Source: CAD feature listing. Evaluate the final solid. Frame: model axes, mm. Face numbers are marked on the shaded views. A direction names the side the tool comes from. Coordinates: 2 decimals unless noted, no trailing zeros. Order: outer loops, then holes, each group sorted by start corner. A loop starts at its lowest first (then second) coordinate and runs counter-clockwise, first axis right, second up. Notation, with made-up numbers: (23, 70.25) - (71, 70.25) arc R3 cw to (71, 74.25) - close; hole circle Ø5 at (64, 30.25). An arc over 180 degrees is marked (long way). One line per question, with ' | ' between items.
from build123d import *

# Parameters (mm, degrees)
BOSS_EXTRUDE1_DEPTH = 15
SKETCH4_R           = 37.5
BOSS_EXTRUDE2_DEPTH = 25
SKETCH5_R           = 22.5
CUT_EXTRUDE1_DEPTH  = 179.290493297
SKETCH6_R           = 32.5
CUT_EXTRUDE2_DEPTH  = 15
SKETCH7_R           = 15
CUT_EXTRUDE3_DEPTH  = 178.165177165
SKETCH9_R           = 15
BOSS_EXTRUDE3_DEPTH = 5
SKETCH10_R          = 1.5
CUT_EXTRUDE7_DEPTH  = 3


with BuildPart() as part:
    # Sketch2 → Boss-Extrude1 (new body)
    with BuildSketch(Plane(origin=(0, 0, 0), x_dir=(1, 0, 0), z_dir=(0, 1, 0))):
        with BuildLine():
            Line((0, 22.5), (150, 22.5))
            ThreePointArc((150, 22.5), (172.5, 0), (150, -22.5))
            Line((150, -22.5), (0, -22.5))
            ThreePointArc((0, -22.5), (-22.5, 0), (0, 22.5))
        make_face()
    extrude(amount=BOSS_EXTRUDE1_DEPTH)

    # Sketch4 → Boss-Extrude2 (add)
    with BuildSketch(Plane(origin=(0, 15, 0), x_dir=(1, 0, 0), z_dir=(0, 1, 0))):
        with Locations(Location((0, 0, 0), (0, 0, 270))):
            Circle(SKETCH4_R)
    extrude(amount=-BOSS_EXTRUDE2_DEPTH)

    # Sketch5 → Cut-Extrude1 (cut, through all)
    with BuildSketch(Plane(origin=(0, 15, 0), x_dir=(1, 0, 0), z_dir=(0, 1, 0))):
        with Locations(Location((0, 0, 0), (0, 0, 270))):
            Circle(SKETCH5_R)
    extrude(amount=-CUT_EXTRUDE1_DEPTH, mode=Mode.SUBTRACT)

    # Sketch6 → Cut-Extrude2 (cut)
    with BuildSketch(Plane(origin=(0, 15, 0), x_dir=(1, 0, 0), z_dir=(0, 1, 0))):
        with Locations(Location((0, 0, 0), (0, 0, 270))):
            Circle(SKETCH6_R)
    extrude(amount=-CUT_EXTRUDE2_DEPTH, mode=Mode.SUBTRACT)

    # Sketch7 → Cut-Extrude3 (cut, through all)
    with BuildSketch(Plane.XZ):
        with Locations(Location((150, 0, 0), (0, 0, 270))):
            Circle(SKETCH7_R)
    extrude(amount=-CUT_EXTRUDE3_DEPTH, mode=Mode.SUBTRACT)

    # Sketch9 → Boss-Extrude3 (add)
    with BuildSketch(Plane.XZ):
        with Locations(Location((150, 0, 0), (0, 0, 270))):
            Circle(SKETCH9_R)
    extrude(amount=-BOSS_EXTRUDE3_DEPTH)

    # Sketch10 → Cut-Extrude7 (cut)
    with BuildSketch(Plane(origin=(0, 15, 0), x_dir=(1, 0, 0), z_dir=(0, 1, 0))):
        with Locations(Location((0, -34.5, 0), (0, 0, 270))):
            Circle(SKETCH10_R)
        with Locations(Location((34.5, 0, 0), (0, 0, 270))):
            Circle(SKETCH10_R)
        with Locations(Location((0, 34.5, 0), (0, 0, 270))):
            Circle(SKETCH10_R)
    extrude(amount=-CUT_EXTRUDE7_DEPTH, mode=Mode.SUBTRACT)


solid = part.part
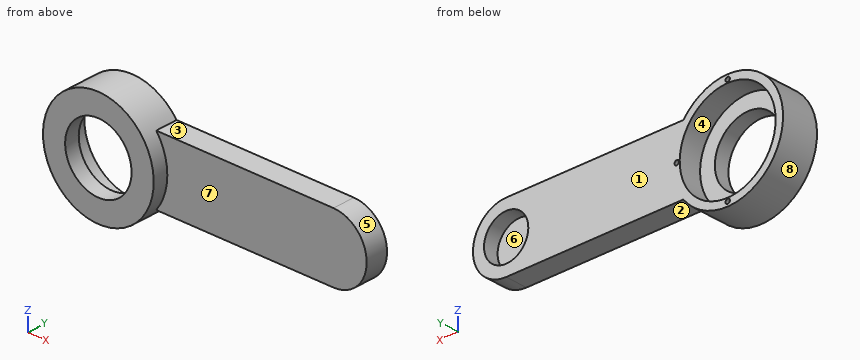
(1) Pin query (flat end, axial travel): P1, Ø12, axis at x = 84, y = 8, coming from the -Z side; P2, Ø3.5, axis at x = -0.5, z = 34.5, coming from the +Y side; P3, Ø22.5, axis at x = 91.5, z = -11, coming from the -Y side; P4, Ø1.5, axis at y = -6, z = 26, coming from the +X side. Return the tip coordinate at first contact, or that it passes through.
Taken from the geometry:
P1: stops at z = -22.5 | P2: stops at y = 15 | P3: stops at y = 0 | P4: stops at x = 27.73
(2) Pull-direction query (X, two-part tool) for the marked faces 6, 7 and 8; classes: pulls with the +X half, pulls with the -X half, needs draft (parallel to the pull), parting line crosses it, or undercut.
Taken from the geometry:
face 6: undercut | face 7: needs draft | face 8: parting line crosses it
(3) Cut plane C-C (x = -14.5). Return the cut outline in (y, z).
Taken from the geometry:
outline: (-10, -34.58) - (15, -34.58) - (15, -29.09) - (0, -29.09) - (0, -17.2) - (-10, -17.2) - close; (-10, 17.2) - (0, 17.2) - (0, 29.09) - (15, 29.09) - (15, 34.58) - (-10, 34.58) - close
(4) Cut plane D-D (y = -3.75). Return the cut outline in (x, z), and give its area (3 significant figures).
Taken from the geometry:
outline: circle Ø75 at (0, 0); hole circle Ø45 at (0, 0) | area: 2,830 mm²
(5) Cut plane B-B (y = 9.25). Return the cut outline in (x, z).
Taken from the geometry:
outline: (30, -22.5) - (150, -22.5) arc R22.5 ccw to (150, 22.5) - (30, 22.5) arc R37.5 ccw (long way) to start; hole circle Ø65 at (0, 0); hole circle Ø30 at (150, 0)
(6) Material intervals for L1, parallel to X at y = 12.75, z = 0; L2, parallel to X at y = 11.5, z = 0; L3, parallel to X at y = 10, z = 4.5, sorted ascending. Write a range as from..to.
Taken from the geometry:
L1: x = -37.5..-32.5, 32.5..33, 36..135, 165..172.5 | L2: x = -37.5..-32.5, 32.5..135, 165..172.5 | L3: x = -37.23..-32.19, 32.19..135.69, 164.31..172.05
(7) Set-up query: the marked faces 1, 2, 3, 4 and 5. Return all of +Z, -Z, +X, -X, +Y, -Y with unobstructed straight access to the full face (end or side cutting, diameter ignored); none if empty.
Taken from the geometry:
face 1: +Z, -Z, +X, -X, +Y | face 2: -Z, +X, +Y, -Y | face 3: +Z, +X, +Y, -Y | face 4: +Y | face 5: +X, +Y, -Y
(8) Cut plane A-A (z = -11.5). Return the cut outline in (x, y).
Taken from the geometry:
outline: (-35.69, -10) - (-19.34, -10) - (-19.34, 0) - (-30.4, 0) - (-30.4, 15) - (-35.69, 15) - close; (19.34, -10) - (35.69, -10) - (35.69, 0) - (169.34, 0) - (169.34, 15) - (159.63, 15) - (159.63, 5) - (140.37, 5) - (140.37, 15) - (30.4, 15) - (30.4, 0) - (19.34, 0) - close
